Answer from the drawing. Dimensions are ordinates in mm from the lowest x, y and z of the part. A direction names the side the tool comes from. Give positions to 0.01 mm unless a question says otherwise; leave off trailing zeros. Loops run counter-clockwise (first coordinate to the right, second up) from the corner with the lowest first, then second, coordinate; pieces in that order, holes last.
Item 1: Section B-B, the plane x = 8.5 is taken. Give the vertices of the cut face in (y, z), and give its area (3 significant figures).
Item 2: Section C-C, the plane x = 19.75 is taken. Give the vertices of the cut face in (y, z), and give its area (3 significant figures).
Item 3: A tool of negligible diameter and unlimited length cuts with its end or side. For the marked faces 1, 2 and 3, from which of +Z, -Z, +X, -X, +Y, -Y can it reach the whole face along a straight path? Write none if from no direction.
Item 4: Consider line 1 along Z through (x, y) = (10, 52); line 2 along Y through (x, z) = (21, 1.75); line 3 along X through (y, z) = (66, 15.95). Determine where each line is inside the solid, lowest interval first.
Item 5: Section A-A, the plane z = 3.5 is taken. Give the vertices of the cut face in (x, y).
Item 6: Section D-D, the plane z = 12.25 is taken. Give the vertices of the cut face in (x, y).
Item 7: Each of these flat-tipped pins is pushed along its axis until it touches: pin 1 Ø3.5 at (y, z) = (6, 11.5) entering from -X; pin 2 Ø5 at (x, z) = (13.5, 4) entering from +Y; pin 3 Ø2 at (x, y) = (13.5, 27) entering from -Z. Where does it stop, or does it pass through?
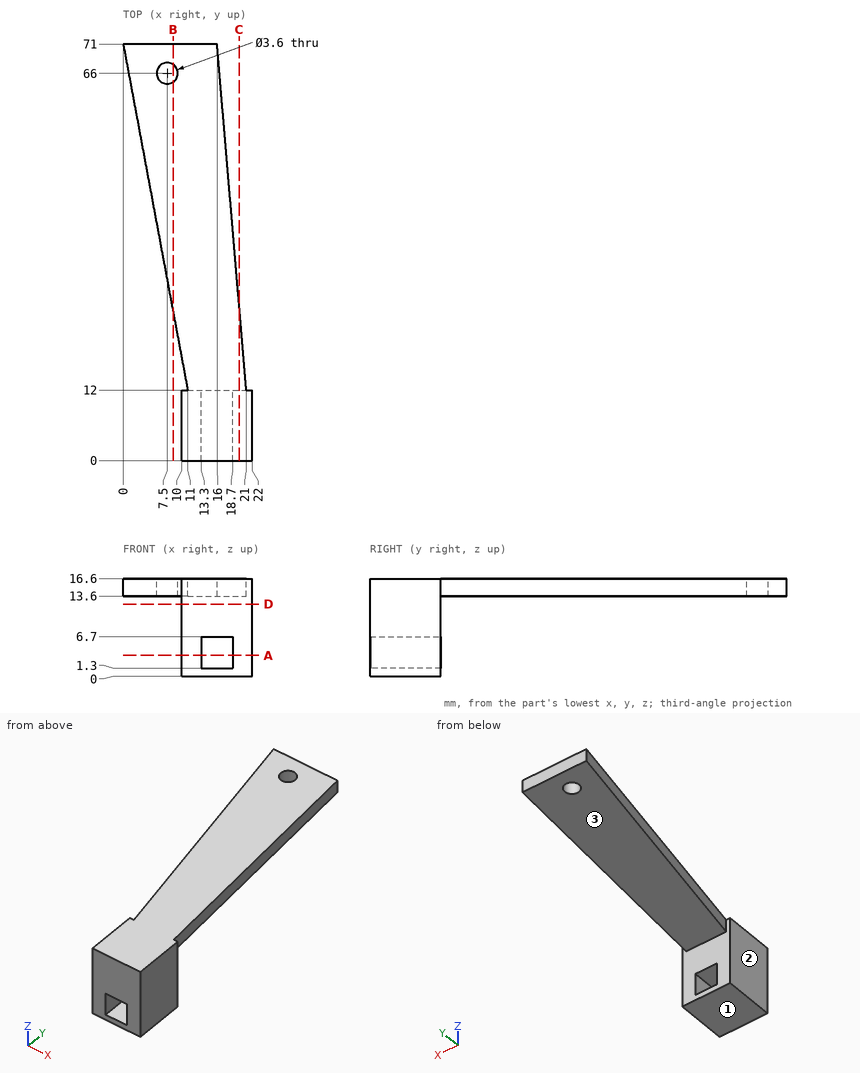
Worked answers:
1. outline: (25.41, 13.6) - (64.5, 13.6) - (64.5, 16.6) - (25.41, 16.6) - close; (67.5, 13.6) - (71, 13.6) - (71, 16.6) - (67.5, 16.6) - close
1. area: 128 mm2
2. outline: (0, 0) - (12, 0) - (12, 13.6) - (26.75, 13.6) - (26.75, 16.6) - (0, 16.6) - close
2. area: 243 mm2
3. face 1: -Z, +X, -X, +Y, -Y
3. face 2: +Z, -Z, -X, -Y
3. face 3: -Z, +X, -X, +Y
4. line 1: z = 13.6 to 16.6
4. line 2: y = 0 to 12
4. line 3: x = 0.93 to 5.7, 9.3 to 16.42
5. outline: (10, 0) - (13.3, 0) - (13.3, 12) - (10, 12) - close; (18.7, 0) - (22, 0) - (22, 12) - (18.7, 12) - close
6. outline: (10, 0) - (22, 0) - (22, 12) - (10, 12) - close
7. pin 1: stops at x = 10
7. pin 2: stops at y = 12
7. pin 3: stops at z = 13.6
